Can you work these out from the drawing? Everything is in mm from the part's minimum corner. Coordinates: 2 decimals unless noted, no trailing zeros. Order: outer loops, then holes, each group sorted by start corner. A loop starts at its lowest first (then second) coordinate and runs counter-clockwise, first axis right, second up. Notation, with made-up numbers: M 65.25,60 L 90.25,60 A27 cw 90.25,90 Z; hole C -14,44.5 d11. An arc over 180 degrees is marked long. Answer as CSV lines item,"result". Start each with the question number.
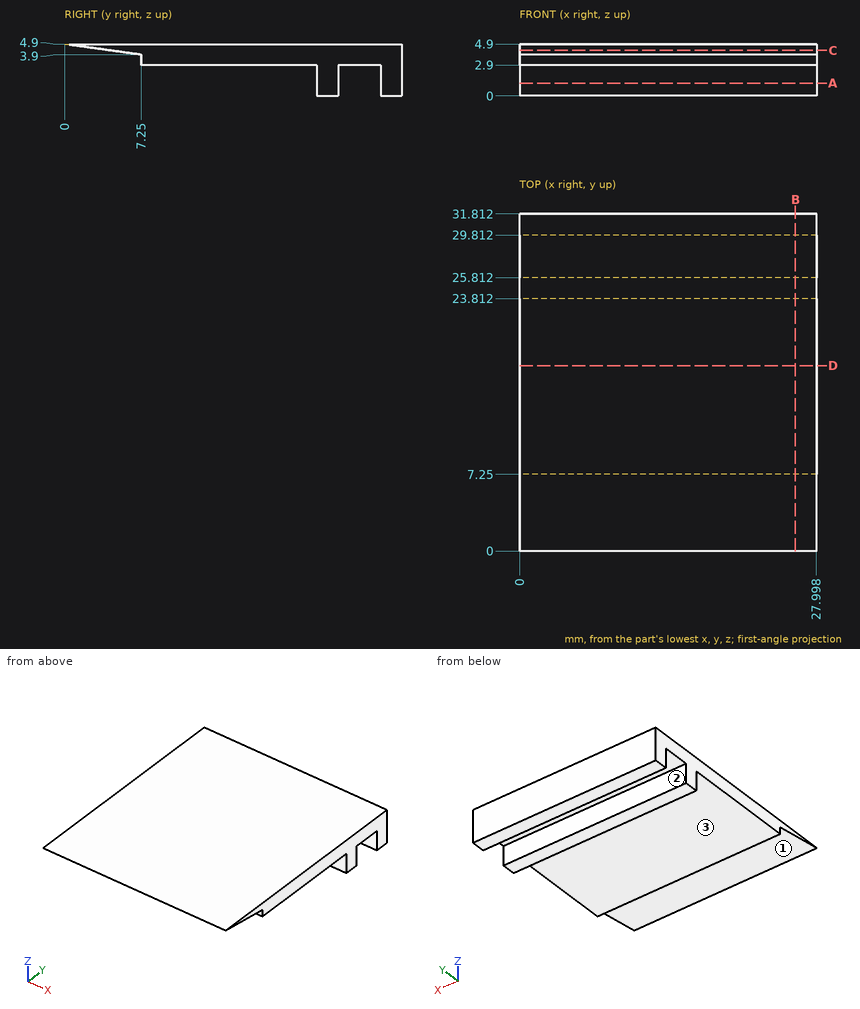
1) I need wall thicknesses on line 1 (Y direction, x = 12.25, z = 1.95); line 2 (Z direction, x = 15, y = 11.5); line 3 (Y direction, x = 2.75, z = 3.15). Which ranges of each line are inside material? Lowest first, please. Write a range as [from, to].
2) Suppose I cut it at C-C on z = 4.3. Please give me the cut outline in (x, y).
3) If we mould it in two halves opening along Y, with no side actions, what happens to the marked faces 1, 2 and 3? For each: released by +Y, released by -Y, zero draft, split by the parting line, or undercut.
4) Suppose I cut it at D-D on y = 17.5. Please give me the cut outline in (x, z).
5) Suppose I cut it at A-A on z = 1.2. Please give me the cut outline in (x, y), plus the area to 3 significant figures.
6) Suppose I cut it at B-B on x = 26. Please give me the cut outline in (y, z).
7) Will these pins go through, and if not, where does the flat tip stop? pin 1 Ø1.5 at (x, z) = (18.5, 2) entering from -Y; pin 2 Ø1.2 at (x, y) = (14.5, 28.5) entering from -Z.
Output:
1,line 1,"[23.81, 25.81], [29.81, 31.81]"
1,line 2,"[2.9, 4.9]"
1,line 3,"[7.25, 31.81]"
2,outline,"M 0,4.35 L 28,4.35 L 28,31.81 L 0,31.81 Z"
3,face 1,"released by -Y"
3,face 2,"undercut"
3,face 3,"zero draft"
4,outline,"M 0,2.9 L 28,2.9 L 28,4.9 L 0,4.9 Z"
5,outline,"M 0,23.81 L 28,23.81 L 28,25.81 L 0,25.81 Z; M 0,29.81 L 28,29.81 L 28,31.81 L 0,31.81 Z"
5,area,"112 mm²"
6,outline,"M 0,4.9 L 7.25,3.9 L 7.25,2.9 L 23.81,2.9 L 23.81,0 L 25.81,0 L 25.81,2.9 L 29.81,2.9 L 29.81,0 L 31.81,0 L 31.81,4.9 Z"
7,pin 1,"y = 23.81"
7,pin 2,"z = 2.9"
